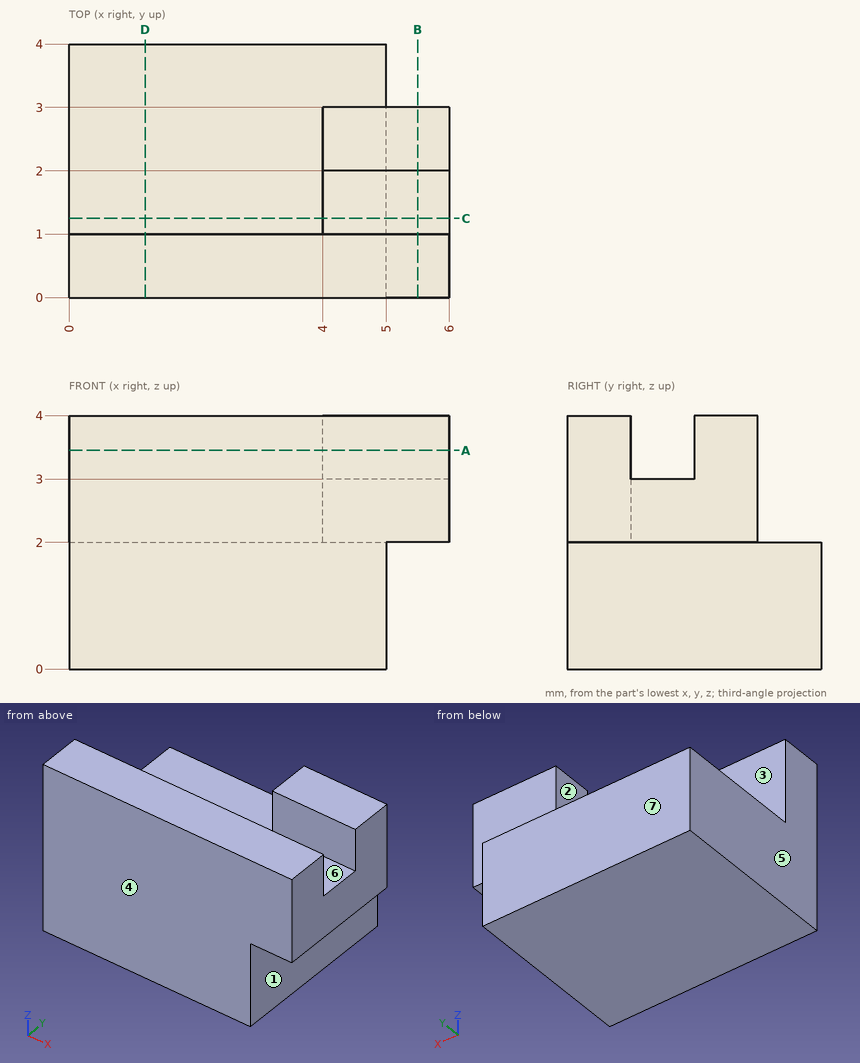
Part print with two shaded views. Sizes in mm from the minimum x, y, z corner. A direction names the side the tool comes from. Round coordinates to 2 decimals unless told otherwise and drop trailing zeros. Order: outer loops, then holes, each group sorted by start corner. A loop starts at its lowest first (then second) coordinate and runs counter-clockwise, first axis right, second up.
(1) Pin check, flat tips, straight feed: pin 1 (2 mm diameter, centred on x = 4.5, z = 3.5, fed in from +Y); pin 2 (0.8 mm diameter, centred on x = 4.5, y = 1.5, fed in from +Z); pin 3 (1.6 mm diameter, centred on y = 3, z = 1, fed in from +X). Stop position of each tip, or through.
(2) Band-saw the part on A-A (z = 3.45). List the corners of the cut face in (x, y), then the cut area to 3 significant figures.
(3) Band-saw the part on B-B (x = 5.5). List the corners of the cut face in (y, z), then the cut area to 3 significant figures.
(4) Band-saw the part on C-C (y = 1.25). List the corners of the cut face in (x, z).
(5) Drill centre lines: line 1 (Y direction, x = 5.25, z = 3.85); line 2 (Y direction, x = 2.15, z = 3.25); line 3 (Z direction, x = 3, y = 3.55). Where is each one in solid material? Low to high.
(6) Band-saw the part on D-D (x = 1.2). List the corners of the cut face in (y, z), then the cut area to 3 significant figures.
(7) Pull direction Y, two halves, no side cores. Call the marked faces 4, 5, 6 and 7: released by +Y, released by -Y, zero draft, split by the parting line, or undercut.
(8) 3-axis set-ups, long thin cutter, end or side, ignore diameter. For the marked faces 1, 2 and 3: which of +Z, -Z, +X, -X, +Y, -Y reach the whole face in a straight line?
Verdict:
1. pin 1: stops at y = 3
1. pin 2: stops at z = 3
1. pin 3: stops at x = 5
2. outline: (0, 0) - (6, 0) - (6, 1) - (0, 1) - close; (4, 2) - (6, 2) - (6, 3) - (4, 3) - close
2. area: 8.00 mm2
3. outline: (0, 2) - (3, 2) - (3, 4) - (2, 4) - (2, 3) - (1, 3) - (1, 4) - (0, 4) - close
3. area: 5.00 mm2
4. outline: (0, 0) - (5, 0) - (5, 2) - (6, 2) - (6, 3) - (4, 3) - (4, 2) - (0, 2) - close
5. line 1: y = 0 to 1, 2 to 3
5. line 2: y = 0 to 1
5. line 3: z = 0 to 2
6. outline: (0, 0) - (4, 0) - (4, 2) - (1, 2) - (1, 4) - (0, 4) - close
6. area: 10.0 mm2
7. face 4: released by -Y
7. face 5: zero draft
7. face 6: undercut
7. face 7: released by +Y
8. face 1: -Z, +X, +Y, -Y
8. face 2: +Z, -X, +Y
8. face 3: +Z, -X
